```python
from build123d import *

# Parameters (mm, degrees)
SKETCH3_W               = 262.8
SKETCH3_H               = 305.28
BOSS_EXTRUDE3_DEPTH     = 10
CUT_EXTRUDE1_DEPTH      = 202.655472527
CUT_EXTRUDE1_DEPTH_BACK = 202.655472527
CUT_EXTRUDE2_DEPTH      = 202.655472527
CUT_EXTRUDE2_DEPTH_BACK = 202.655472527
SKETCH5_R               = 36
SKETCH6_R               = 20.52
BOSS_EXTRUDE4_DEPTH     = 125
CUT_EXTRUDE3_DEPTH      = 243.466347356
CUT_EXTRUDE3_DEPTH_BACK = 243.466347356
SKETCH7_R               = 17.5


with BuildPart() as part:
    # Sketch3 → Boss-Extrude3 (new body)
    with BuildSketch(Plane(origin=(0, 0, 0), x_dir=(1, 0, 0), z_dir=(0, 1, 0))):
        Rectangle(SKETCH3_W, SKETCH3_H)
    extrude(amount=BOSS_EXTRUDE3_DEPTH)

    # Sketch4 → Cut-Extrude1 (cut, two sides: drawn at the far end of the back side and taken through both)
    with BuildSketch(Plane(origin=(0, 10, 0), x_dir=(1, 0, 0), z_dir=(0, 1, 0)).offset(-CUT_EXTRUDE1_DEPTH_BACK)):
        with BuildLine():
            Line((-131.4, -90), (-131.4, -152.64))
            Line((-131.4, -152.64), (-70.92, -152.64))
            ThreePointArc((-70.92, -152.64), (-107.755247271, -127.687824951), (-131.4, -90))
        make_face()
        with BuildLine():
            Line((83.16, -152.64), (131.4, -152.64))
            Line((131.4, -152.64), (131.4, -72.72))
            ThreePointArc((131.4, -72.72), (117.938305095, -119.113391364), (83.16, -152.64))
        make_face()
        with BuildLine():
            Line((-99.372734155, 121.287125755), (-67.345468311, 121.287125755))
            Line((-67.345468311, 121.287125755), (-48.15934209, 152.64))
            Line((-48.15934209, 152.64), (-131.4, 152.64))
            Line((-131.4, 152.64), (-131.4, 83.52))
            ThreePointArc((-131.4, 83.52), (-119.737831056, 106.093689962), (-99.372734155, 121.287125755))
        make_face()
        with BuildLine():
            Line((131.4, 83.52), (131.4, 152.64))
            Line((131.4, 152.64), (62.28, 152.64))
            ThreePointArc((62.28, 152.64), (109.286007047, 130.526007047), (131.4, 83.52))
        make_face()
    extrude(amount=CUT_EXTRUDE1_DEPTH + CUT_EXTRUDE1_DEPTH_BACK, mode=Mode.SUBTRACT)

    # Sketch5 → Cut-Extrude2 (cut, two sides: drawn at the far end of the back side and taken through both)
    with BuildSketch(Plane(origin=(0, 10, 0), x_dir=(1, 0, 0), z_dir=(0, 1, 0)).offset(-CUT_EXTRUDE2_DEPTH_BACK)):
        with Locations(Location((0, 0, 0), (0, 0, 270))):
            Circle(SKETCH5_R)
    extrude(amount=CUT_EXTRUDE2_DEPTH + CUT_EXTRUDE2_DEPTH_BACK, mode=Mode.SUBTRACT)

    # Sketch6 → Boss-Extrude4 (add)
    with BuildSketch(Plane(origin=(0, 10, 0), x_dir=(1, 0, 0), z_dir=(0, 1, 0))):
        with Locations(Location((0, 95.04, 0), (0, 0, 90))):
            Circle(SKETCH6_R)
        with Locations(Location((0, -95.04, 0), (0, 0, 90))):
            Circle(SKETCH6_R)
    extrude(amount=BOSS_EXTRUDE4_DEPTH)

    # Sketch7 → Cut-Extrude3 (cut, two sides: drawn at the far end of the back side and taken through both)
    with BuildSketch(Plane(origin=(0, 135, 0), x_dir=(1, 0, 0), z_dir=(0, 1, 0)).offset(-CUT_EXTRUDE3_DEPTH_BACK)):
        with Locations(Location((0, 95.04, 0), (0, 0, 270))):
            Circle(SKETCH7_R)
        with Locations(Location((0, -95.04, 0), (0, 0, 90))):
            Circle(SKETCH7_R)
    extrude(amount=CUT_EXTRUDE3_DEPTH + CUT_EXTRUDE3_DEPTH_BACK, mode=Mode.SUBTRACT)


solid = part.part
```
Work out the finished part from the listing and answer in its coordinate system (mm). A direction names the side the tool comes from. Round coordinates to 2 decimals unless told otherwise and drop trailing zeros. Loops run counter-clockwise (first coordinate to the right, second up) from the corner with the lowest first, then second, coordinate; pieces in that order, holes last.
(1) The part is cut by section A-A, the plane z = 0. Give the vertices of the cut face in (x, y), and give its area (3 significant figures).
Computed values:
outline: (-131.4, 0) - (-36, 0) - (-36, 10) - (-131.4, 10) - close; (36, 0) - (131.4, 0) - (131.4, 10) - (36, 10) - close
area: 1,910 mm2
(2) Each of these flat-tipped pins is pushed along its axis until it touches: P1, Ø5, axis at x = -5.5, y = 84.5, coming from the -Z side; P2, Ø1, axis at x = -81, z = 107.5, coming from the +Y side; P3, Ø11, axis at x = -83.5, y = 7, coming from the -Z side. Where does it stop, or does it pass through?
Computed values:
P1: stops at z = -115.34
P2: stops at y = 10
P3: stops at z = -121.29
(3) For faces 1 (the cylindrical face through (-0.9, 71.62, 115.54)), 2 (the flat face through (-84, 5, -121.287)), 3 (the cylindrical face through (0.769, 66.555, -112.523)), determine the directions among +Z, -Z, +X, -X, +Y, -Y from which every point of the face is accessible in a straight line to the end or side of a thin tool.
Computed values:
face 1: +Y
face 2: -Z, -X, +Y, -Y
face 3: +Y, -Y
(4) The part is cut by section C-C, the plane y = 15.5. Give the vertices of the cut face in (x, z), and give its area (3 significant figures).
Computed values:
outline: circle Ø41.04 at (0, -95.04); circle Ø41.04 at (0, 95.04); hole circle Ø35 at (0, -95.04); hole circle Ø35 at (0, 95.04)
area: 721 mm2
(5) The part is cut by section D-D, the plane z = 66. Give the vertices of the cut face in (x, y), and give its area (3 significant figures).
Computed values:
outline: (-131.4, 0) - (131.4, 0) - (131.4, 10) - (-131.4, 10) - close
area: 2,630 mm2
(6) The mould has two halves that part along X. Classify faces 4 (the flat face through (131.4, 5, -4)), 5 (the flat face through (-9.22, 135, -110.14)), 6 (the cylindrical face through (-0.769, 66.555, 112.523)): pulls with the +X half, pulls with the -X half, needs draft (parallel to the pull), parting line crosses it, or undercut.
Computed values:
face 4: pulls with the +X half
face 5: needs draft
face 6: undercut
(7) The part is cut by section B-B, the plane x = 0. Give the vertices of the cut face in (y, z), and give its area (3 significant figures).
Computed values:
outline: (0, -152.64) - (10, -152.64) - (10, -115.56) - (135, -115.56) - (135, -112.54) - (0, -112.54) - close; (0, -77.54) - (135, -77.54) - (135, -74.52) - (10, -74.52) - (10, -36) - (0, -36) - close; (0, 36) - (10, 36) - (10, 74.52) - (135, 74.52) - (135, 77.54) - (0, 77.54) - close; (0, 112.54) - (135, 112.54) - (135, 115.56) - (10, 115.56) - (10, 152.64) - (0, 152.64) - close
area: 3,140 mm2
(8) Find the intervals of material crossed by L1, parallel to X at y = 91, z = -95; L2, parallel to Y at x = 47, z = -5; L3, parallel to X at y = 114, z = 103.5, in increasing order.
Computed values:
L1: x = -20.52 to -17.5, 17.5 to 20.52
L2: y = 0 to 10
L3: x = -18.69 to -15.32, 15.32 to 18.69
